Verification items for the finished model (mm, model axes). A direction names the side the tool comes from. Coordinates: 2 decimals unless noted, no trailing zeros. Order: outer loops, then holes, each group sorted by start corner. A loop starts at its lowest first (then second) coordinate and runs counter-clockwise, first axis right, second up. Notation, with made-up numbers: (-18.5, 12) - (0.5, 12) arc R16 ccw to (0.5, 28) - close; hole circle Ø5 at (83.25, -16). An arc over 180 degrees is marked (long way). Answer as CSV lines item,"result". Start each with the question number.
1. Section check B-B (x = -23). Record the cut outline in (y, z), and give its area (3 significant figures).
2. Section check A-A (z = -8.5). Record the cut outline in (x, y).
3. Material ranges on L1, parallel to Z at x = -37.5, y = 0.7; L2, parallel to Z at x = 3, y = 0.15; L3, parallel to X at y = 1.05, z = 36 (3 decimals), recorded low to high. Write a range as [from, to].
4. Go/stop test with flat-tipped pins: pin 1 (1 mm diameter, centred on x = -56, y = 0, fed in from -Z); pin 2 (0.7 mm diameter, centred on y = -1, z = -2.5, fed in from -X); pin 3 (0.5 mm diameter, centred on y = 1, z = -34.5, fed in from +X); pin 4 (8 mm diameter, centred on x = -17.5, z = -23.5, fed in from +Y). Record where each tip stops, or that it passes through.
5. Mould release check, pull along Z, two halves, no side actions. Record for faces 6 (the flat face through (73.871, 1.014, -27.075)), 7 (the flat face through (84, 1, -1.67)), 8 (the flat face through (71.6, 1, -20.2)): pulls with the +Z half, pulls with the -Z half, needs draft (parallel to the pull), parting line crosses it, or undercut.
6. Set-up check for faces 1 (the flat face through (-55, 1, -33.563)), 2 (the flat face through (71.425, 1.014, 15.539)), 3 (the cylindrical face through (-57.04, 1.29, -32.55)), 4 (the flat face through (-55, 1, -31.563)), 5 (the flat face through (84, 1, -3.67)): record each of +Z, -Z, +X, -X, +Y, -Y from which the full face is reachable in a straight line by a thin tool's end or side.
from build123d import *

# Parameters (mm, degrees)
BOSS_EXTRUDE1_DEPTH = 2
EDGE_FLANGE1_DEPTH  = 2
EDGE_FLANGE2_DEPTH  = 2
CUT_EXTRUDE3_DEPTH  = 10


# Sheet-metal steps are written as plain solids
with BuildPart() as part:
    # Sketch2 → Boss-Extrude1 (new body)
    with BuildSketch(Plane(origin=(0, 0, 0), x_dir=(1, 0, 0), z_dir=(0, 1, 0))):
        Polygon((81.609993248, 1.669814581), (81.609993248, -16.836643227), (75.909994488, -22.536641987), (75.909994488, -38.936642207), (70.009993588, -44.836643107), (58.109994528, -44.836643107), (58.109994528, -34.336641247), (63.809993288, -34.336641247), (67.509993508, -30.636641027), (67.509993508, -19.345596807), (75.109993548, -11.745596767), (75.109993548, 16.463358753), (67.709993108, 23.863356653), (67.709993108, 26.763358473), (64.309994828, 30.163356753), (-43.190006072, 30.163356753), (-52.793309772, 30.163356753), (-52.793309772, 31.563357033), (-54.793309772, 31.563357033), (-54.793309772, 33.563357033), (-52.793309772, 33.563357033), (-52.793309772, 34.963357313), (-43.190006072, 34.963357313), (66.209993568, 34.963357313), (81.609993248, 19.563357633), (81.609993248, 3.669814581), (83.609993248, 3.669814581), (83.609993248, 1.669814581), align=None)
    extrude(amount=BOSS_EXTRUDE1_DEPTH)

    # Edge-Flange1 section (across the edge) → Edge-Flange1 (add)
    with BuildSketch(Plane(origin=(-55.793309772, 0, -31.563357033), x_dir=(1, 0, 0), z_dir=(0, 0, -1))):
        with BuildLine():
            Line((-2, 0.5), (-2, 1.4))
            Line((-2, 1.4), (0, 1.4))
            Line((0, 1.4), (0, 0.5))
            ThreePointArc((0, 0.5), (0.146446609, 0.146446609), (0.5, 0))
            Line((0.5, 0), (1, 0))
            Line((1, 0), (1, -2))
            Line((1, -2), (0.5, -2))
            ThreePointArc((0.5, -2), (-1.267766953, -1.267766953), (-2, 0.5))
        make_face()
    extrude(amount=EDGE_FLANGE1_DEPTH)

    # Edge-Flange2 section (across the edge) → Edge-Flange2 (add)
    with BuildSketch(Plane(origin=(84.609993248, 0, -3.669814581), x_dir=(-1, 0, 0), z_dir=(0, 0, 1))):
        with BuildLine():
            Line((-2, 0.5), (-2, 1.4))
            Line((-2, 1.4), (0, 1.4))
            Line((0, 1.4), (0, 0.5))
            ThreePointArc((0, 0.5), (0.146446609, 0.146446609), (0.5, 0))
            Line((0.5, 0), (1, 0))
            Line((1, 0), (1, -2))
            Line((1, -2), (0.5, -2))
            ThreePointArc((0.5, -2), (-1.267766953, -1.267766953), (-2, 0.5))
        make_face()
    extrude(amount=EDGE_FLANGE2_DEPTH)

    # Sketch13 → Cut-Extrude3 (cut)
    with BuildSketch(Plane(origin=(0, 2, 0), x_dir=(1, 0, 0), z_dir=(0, 1, 0))):
        Polygon((64.364993832, 30.231358373), (-43.077006168, 30.231358373), (-52.793309772, 30.231358373), (-52.793309772, 30.163356753), (64.309994828, 30.163356753), (67.709993108, 26.763358473), (67.709993108, 23.863356653), (75.109993548, 16.463358753), (75.109993548, -11.745596767), (67.509993508, -19.345596807), (67.509993508, -30.636641027), (63.809993288, -34.336641247), (58.109994528, -34.336641247), (58.109994528, -44.836643107), (70.009993588, -44.836643107), (75.909994488, -38.936642207), (75.909994488, -22.536641987), (81.609993248, -16.836643227), (81.609993248, 1.669814581), (81.509993832, 1.669814581), (81.509993832, -16.758641627), (75.794993832, -22.473641627), (75.794993832, -38.856641627), (71.222993832, -43.428641627), (58.268993832, -43.428641627), (58.268993832, -35.554641627), (65.126993832, -35.554641627), (67.665284412, -33.016351047), (67.669899592, -19.298575587), (75.286993832, -11.672504987), (75.286993832, 16.515358373), (67.793993832, 24.008355833), (67.793993832, 26.802358373), align=None)
        Polygon((-52.793309772, 30.163356753), (-52.793309772, 30.231358373), (-53.09278865, 30.231358373), (-53.09278865, 29.122247983), (64.073173088, 29.122247983), (66.904295046, 26.802358373), (66.904295046, 23.685270997), (74.890508664, 15.670381273), (73.855495628, -9.951608799), (66.571415804, -17.811521066), (66.392045366, -24.291741654), (65.126993832, -32.125935595), (57.650093481, -33.249786732), (57.276841603, -46.73447534), (58.268993832, -46.73447534), (69.513593476, -46.73447534), (76.944541222, -41.148796497), (77.641700893, -23.890445583), (84.109993248, -17.212504202), (84.109993248, 1.669814581), (81.609993248, 1.669814581), (81.609993248, -16.836643227), (75.909994488, -22.536641987), (75.909994488, -38.936642207), (70.009993588, -44.836643107), (58.109994528, -44.836643107), (58.109994528, -34.336641247), (63.809993288, -34.336641247), (67.509993508, -30.636641027), (67.509993508, -19.345596807), (75.109993548, -11.745596767), (75.109993548, 16.463358753), (67.709993108, 23.863356653), (67.709993108, 26.763358473), (64.309994828, 30.163356753), align=None)
        Polygon((84.109993248, 19.032357692), (84.109993248, 3.669814581), (81.509993832, 3.669814581), (81.509993832, 19.436358373), (66.015993832, 34.930358373), (62.967993832, 34.930358373), (62.967993832, 33.914358373), (60.681993832, 33.914358373), (60.681993832, 34.930358373), (48.489993832, 34.930358373), (48.489993832, 33.914358373), (46.203993832, 33.914358373), (46.203993832, 34.930358373), (33.376993832, 34.930358373), (33.376993832, 33.914358373), (30.963993832, 33.914358373), (30.963993832, 34.930358373), (18.644993832, 34.930358373), (18.644993832, 33.914358373), (16.358993832, 33.914358373), (16.358993832, 34.930358373), (3.912993832, 34.930358373), (3.912993832, 33.914358373), (1.499993832, 33.914358373), (1.499993832, 34.930358373), (-11.327006168, 34.930358373), (-11.327006168, 33.914358373), (-13.740006168, 33.914358373), (-13.740006168, 34.930358373), (-26.567006168, 34.930358373), (-26.567006168, 33.914358373), (-28.980006168, 33.914358373), (-28.980006168, 34.930358373), (-41.172006168, 34.930358373), (-41.172006168, 33.914358373), (-44.172006168, 33.914358373), (-44.172006168, 34.930358373), (-54.307784522, 34.930358373), (-54.307784522, 35.697895733), (66.904295046, 35.697895733), align=None)
    extrude(amount=-CUT_EXTRUDE3_DEPTH, mode=Mode.SUBTRACT)


solid = part.part
Evaluation:
1,outline,"(0, -34.93) - (2, -34.93) - (2, -30.23) - (0, -30.23) - close"
1,area,"9.40 mm²"
2,outline,"(75.29, 0) - (81.51, 0) - (81.51, 2) - (75.29, 2) - close"
3,L1,"z = [-34.93, -30.23]"
3,L2,"z = [-33.91, -30.23]"
3,L3,"x = [58.269, 75.795]"
4,pin 1,"stops at z = -33.56"
4,pin 2,"stops at x = 84.61"
4,pin 3,"stops at x = 66.7"
4,pin 4,"passes through"
5,face 6,"pulls with the -Z half"
5,face 7,"pulls with the +Z half"
5,face 8,"undercut"
6,face 1,"-Z, -X, +Y, -Y"
6,face 2,"-X, +Y, -Y"
6,face 3,"+Z, -Z, -X, +Y"
6,face 4,"+Z, -X, +Y, -Y"
6,face 5,"-Z, +X, +Y, -Y"
